Model file for the job. Use its own axes, mm. Face numbers are marked on the shaded views. A direction names the side the tool comes from. Give positions to 0.01 mm unless a question says otherwise; leave off trailing zeros. Order: outer loops, then holes, each group sorted by start corner. A loop starts at its lowest first (then second) coordinate and runs counter-clockwise, first axis right, second up. Notation, with made-up numbers: (44, 75) - (76, 75) arc R37 cw to (76, 111) - close; hole circle Ø5 at (65.5, 21.25). An arc over 180 degrees is marked (long way). Use CSV: the item, a comma, the result in double quotes. Start each with the question number.
(1) Drop flat-ended pins along their axis: pin 1 Ø2 at (y, z) = (35, 10.5) entering from -X; pin 2 Ø1.5 at (x, z) = (592, 18) entering from +Y; pin 3 Ø2 at (x, z) = (570, 10) entering from +Y. Give the stop position or say it passes through.
(2) Band-saw the part on C-C, the plane y = 49.5. Give the cut face in (x, z), then the cut area to 3 significant figures.
(3) Band-saw the part on D-D, the plane z = 10. Count the separate pieces of the cut face and the enclosed holes in it, then the cut area to 3 significant figures.
(4) Probe L1, parallel to Y at x = 582, z = 4.75; L2, parallel to Y at x = 574.5, z = 6.5; L3, parallel to Y at x = 594, z = 14. List the from-to ranges inside material, lowest first.
(5) Tool access for the marked faces 4, 5 and 6: list every direction of +Z, -Z, +X, -X, +Y, -Y with a clear straight run to the whole face (end or side of a thin tool).
(6) Band-saw the part on A-A, the plane x = 588. Give the cut face in (y, z), then the cut area to 3 significant figures.
(7) Pull direction Y, two halves, no side cores. Call the marked faces 1, 2 and 3: +Y half, -Y half, draft (parallel to the pull), parting line (faces both ways), or undercut.
(8) Band-saw the part on B-B, the plane y = 63. Give the cut face in (x, z), then the cut area to 3 significant figures.
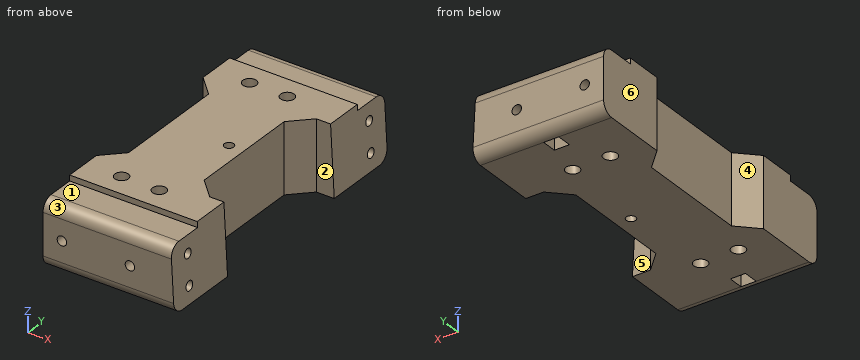
from build123d import *

# Parameters (mm, degrees)
CYLINDER445_R          = 1.25
CYLINDER445_DEPTH      = 20
BOX297_W               = 4
BOX297_H               = 4
BOX297_DEPTH           = 5
BOX298_W               = 4
BOX298_H               = 4
BOX298_DEPTH           = 5
CYLINDER444_R          = 1.25
CYLINDER444_DEPTH      = 15
CYLINDER443_R          = 1.25
CYLINDER443_DEPTH      = 15
CYLINDER442_R          = 1.25
CYLINDER442_DEPTH      = 15
CYLINDER441_R          = 1.25
CYLINDER441_DEPTH      = 15
CYLINDER450_R          = 1.8
CYLINDER450_DEPTH      = 18.5
CYLINDER451_R          = 1.8
CYLINDER451_DEPTH      = 18.5
CYLINDER446_R          = 1.8
CYLINDER446_DEPTH      = 18.5
CYLINDER447_R          = 1.8
CYLINDER447_DEPTH      = 18.5
CYLINDER449_R          = 1.25
CYLINDER449_DEPTH      = 15
CYLINDER448_R          = 1.25
CYLINDER448_DEPTH      = 15
CYLINDER440_R          = 1.25
CYLINDER440_DEPTH      = 15
CYLINDER439_R          = 1.25
CYLINDER439_DEPTH      = 15
BOX293_W               = 10
BOX293_H               = 82
BOX293_DEPTH           = 32
BOX293_PLACEMENT_ANGLE = 3
BOX300_W               = 35
BOX300_H               = 10
BOX300_DEPTH           = 1.5
BOX295_W               = 35
BOX295_H               = 20
BOX295_DEPTH           = 17
BOX292_W               = 35
BOX292_H               = 20
BOX292_DEPTH           = 17
BOX296_W               = 20
BOX296_H               = 40
BOX296_DEPTH           = 18.5
BOX299_W               = 35
BOX299_H               = 10
BOX299_DEPTH           = 1.5
FILLET107_R            = 3
CHAMFER030_SIZE        = 4.99


with BuildPart() as cylinder445:
    # Cylinder445 → Cylinder445 (new body)
    with BuildSketch(Plane(origin=(586, 31, 1.5), x_dir=(1, 0, 0), z_dir=(0, 0, 1))):
        Circle(CYLINDER445_R)
    extrude(amount=CYLINDER445_DEPTH)


with BuildPart() as box297:
    # Box297 → Box297 (new body)
    with BuildSketch(Plane(origin=(579, -6, 1.5), x_dir=(1, 0, 0), z_dir=(0, 0, 1))):
        with Locations((2, 2)):
            Rectangle(BOX297_W, BOX297_H)
    extrude(amount=BOX297_DEPTH)


with BuildPart() as fusion398:
    # Box298 → Box298 (new body)
    with BuildSketch(Plane(origin=(579, 64, 1.5), x_dir=(1, 0, 0), z_dir=(0, 0, 1))):
        with Locations((2, 2)):
            Rectangle(BOX298_W, BOX298_H)
    extrude(amount=BOX298_DEPTH)

    # Fusion398: union Box297
    add(box297.part)


with BuildPart() as cylinder444:
    # Cylinder444 → Cylinder444 (new body)
    with BuildSketch(Plane(origin=(585, 7, 6), x_dir=(0, 0, -1), z_dir=(1, 0, 0))):
        Circle(CYLINDER444_R)
    extrude(amount=CYLINDER444_DEPTH)


with BuildPart() as fusion396:
    # Cylinder443 → Cylinder443 (new body)
    with BuildSketch(Plane(origin=(585, 7, 14), x_dir=(0, 0, -1), z_dir=(1, 0, 0))):
        Circle(CYLINDER443_R)
    extrude(amount=CYLINDER443_DEPTH)

    # Fusion396: union Cylinder444
    add(cylinder444.part)


with BuildPart() as fusion396_1:
    # Fusion396 placement: moved
    add(fusion396.part.moved(Location((0, 58, 0))))


with BuildPart() as cylinder442:
    # Cylinder442 → Cylinder442 (new body)
    with BuildSketch(Plane(origin=(585, 7, 6), x_dir=(0, 0, -1), z_dir=(1, 0, 0))):
        Circle(CYLINDER442_R)
    extrude(amount=CYLINDER442_DEPTH)


with BuildPart() as fusion397:
    # Cylinder441 → Cylinder441 (new body)
    with BuildSketch(Plane(origin=(585, 7, 14), x_dir=(0, 0, -1), z_dir=(1, 0, 0))):
        Circle(CYLINDER441_R)
    extrude(amount=CYLINDER441_DEPTH)

    # Fusion395: union Cylinder442
    add(cylinder442.part)


with BuildPart() as fusion397_1:
    # Fusion395 placement: moved
    add(fusion397.part.moved(Location((0, -10, 0))))

    # Fusion397: union Fusion396
    add(fusion396_1.part)


with BuildPart() as cylinder450:
    # Cylinder450 → Cylinder450 (new body)
    with BuildSketch(Plane(origin=(584, 7, 10.5), x_dir=(1, 0, 0), z_dir=(0, 0, 1))):
        Circle(CYLINDER450_R)
    extrude(amount=CYLINDER450_DEPTH)


with BuildPart() as fusion403:
    # Cylinder451 → Cylinder451 (new body)
    with BuildSketch(Plane(origin=(584, 55, 10.5), x_dir=(1, 0, 0), z_dir=(0, 0, 1))):
        Circle(CYLINDER451_R)
    extrude(amount=CYLINDER451_DEPTH)

    # Fusion403: union Cylinder450
    add(cylinder450.part)


with BuildPart() as fusion403_1:
    # Fusion403 placement: moved
    add(fusion403.part.moved(Location((-9.5, 0, -9))))


with BuildPart() as cylinder446:
    # Cylinder446 → Cylinder446 (new body)
    with BuildSketch(Plane(origin=(584, 7, 10.5), x_dir=(1, 0, 0), z_dir=(0, 0, 1))):
        Circle(CYLINDER446_R)
    extrude(amount=CYLINDER446_DEPTH)


with BuildPart() as fusion405:
    # Cylinder447 → Cylinder447 (new body)
    with BuildSketch(Plane(origin=(584, 55, 10.5), x_dir=(1, 0, 0), z_dir=(0, 0, 1))):
        Circle(CYLINDER447_R)
    extrude(amount=CYLINDER447_DEPTH)

    # Fusion399: union Cylinder446
    add(cylinder446.part)


with BuildPart() as fusion405_1:
    # Fusion399 placement: moved
    add(fusion405.part.moved(Location((0.5, 0, -9))))

    # Fusion405: union Fusion403
    add(fusion403_1.part)


with BuildPart() as cylinder449:
    # Cylinder449 → Cylinder449 (new body)
    with BuildSketch(Plane(origin=(588, 71, 10), x_dir=(1, 0, 0), z_dir=(0, -1, 0))):
        Circle(CYLINDER449_R)
    extrude(amount=CYLINDER449_DEPTH)


with BuildPart() as fusion401:
    # Cylinder448 → Cylinder448 (new body)
    with BuildSketch(Plane(origin=(588, 6, 10), x_dir=(1, 0, 0), z_dir=(0, -1, 0))):
        Circle(CYLINDER448_R)
    extrude(amount=CYLINDER448_DEPTH)

    # Fusion401: union Cylinder449
    add(cylinder449.part)


with BuildPart() as fusion401_1:
    # Fusion401 placement: moved
    add(fusion401.part.moved(Location((-18, 0, 0))))


with BuildPart() as cylinder440:
    # Cylinder440 → Cylinder440 (new body)
    with BuildSketch(Plane(origin=(588, 71, 10), x_dir=(1, 0, 0), z_dir=(0, -1, 0))):
        Circle(CYLINDER440_R)
    extrude(amount=CYLINDER440_DEPTH)


with BuildPart() as fusion404:
    # Cylinder439 → Cylinder439 (new body)
    with BuildSketch(Plane(origin=(588, 6, 10), x_dir=(1, 0, 0), z_dir=(0, -1, 0))):
        Circle(CYLINDER439_R)
    extrude(amount=CYLINDER439_DEPTH)

    # Fusion394: union Cylinder440
    add(cylinder440.part)

    # Fusion404: union Fusion401
    add(fusion401_1.part)


with BuildPart() as box293:
    # Box293 → Box293 (new body)
    with BuildSketch(Plane.XY):
        with Locations((5, 41)):
            Rectangle(BOX293_W, BOX293_H)
    extrude(amount=BOX293_DEPTH)


with BuildPart() as box293_1:
    # Box293 placement: moved
    add(box293.part.moved(Location((600, -10, -3.6))).rotate(Axis((600, -10, -3.6), (0, -1, 0)), BOX293_PLACEMENT_ANGLE))


with BuildPart() as box300:
    # Box300 → Box300 (new body)
    with BuildSketch(Plane(origin=(565, 1, 18.5), x_dir=(1, 0, 0), z_dir=(0, 0, 1))):
        with Locations((17.5, 5)):
            Rectangle(BOX300_W, BOX300_H)
    extrude(amount=BOX300_DEPTH)


with BuildPart() as box295:
    # Box295 → Box295 (new body)
    with BuildSketch(Plane(origin=(565, 51, 1.5), x_dir=(1, 0, 0), z_dir=(0, 0, 1))):
        with Locations((17.5, 10)):
            Rectangle(BOX295_W, BOX295_H)
    extrude(amount=BOX295_DEPTH)


with BuildPart() as box292:
    # Box292 → Box292 (new body)
    with BuildSketch(Plane(origin=(565, -9, 1.5), x_dir=(1, 0, 0), z_dir=(0, 0, 1))):
        with Locations((17.5, 10)):
            Rectangle(BOX292_W, BOX292_H)
    extrude(amount=BOX292_DEPTH)


with BuildPart() as box296:
    # Box296 → Box296 (new body)
    with BuildSketch(Plane(origin=(570, 11, 1.5), x_dir=(1, 0, 0), z_dir=(0, 0, 1))):
        with Locations((10, 20)):
            Rectangle(BOX296_W, BOX296_H)
    extrude(amount=BOX296_DEPTH)


with BuildPart() as rear_cross_member_wide:
    # Box299 → Box299 (new body)
    with BuildSketch(Plane(origin=(565, 51, 18.5), x_dir=(1, 0, 0), z_dir=(0, 0, 1))):
        with Locations((17.5, 5)):
            Rectangle(BOX299_W, BOX299_H)
    extrude(amount=BOX299_DEPTH)

    # Fusion402: union Box300, Box295, Box292, Box296
    add(box300.part)
    add(box295.part)
    add(box292.part)
    add(box296.part)

    # Cut293: cut Box293
    add(box293_1.part, mode=Mode.SUBTRACT)

    # Cut294: cut Fusion404
    add(fusion404.part, mode=Mode.SUBTRACT)

    # Cut295: cut Fusion405
    add(fusion405_1.part, mode=Mode.SUBTRACT)

    # Fillet107
    fillet107_edges = [rear_cross_member_wide.edges().sort_by_distance(p)[0] for p in [
        (582.36636, 71, 1.5),
        (581.920894, 71, 18.5),
        (582.36636, -9, 1.5),
        (581.920894, -9, 18.5),
    ]]
    fillet(fillet107_edges, radius=FILLET107_R)

    # Chamfer030
    chamfer030_edges = [rear_cross_member_wide.edges().sort_by_distance(p)[0] for p in [
        (570, 51, 10.75),
        (590, 51, 10.75),
        (570, 11, 10.75),
        (590, 11, 10.75),
    ]]
    chamfer(chamfer030_edges, length=CHAMFER030_SIZE)

    # Cut296: cut Fusion397
    add(fusion397_1.part, mode=Mode.SUBTRACT)

    # Cut297: cut Fusion398
    add(fusion398.part, mode=Mode.SUBTRACT)

    # Cut298: cut Cylinder445
    add(cylinder445.part, mode=Mode.SUBTRACT)


solid = rear_cross_member_wide.part
Answer block:
1,pin 1,"stops at x = 570"
1,pin 2,"stops at y = 70.44"
1,pin 3,"stops at y = 56"
2,outline,"(566.51, 1.5) - (593.49, 1.5) - (593.49, 20) - (566.51, 20) - close"
2,area,"499 mm2"
3,separate pieces,"1"
3,enclosed holes,"5"
3,area,"2,030 mm2"
4,L1,"y = -9 to -6, -2 to 64, 68 to 71"
4,L2,"y = -9 to 5.2, 8.8 to 53.2, 56.8 to 71"
4,L3,"y = -9 to -4.25, -1.75 to 11.99, 50.01 to 63.75, 66.25 to 71"
5,face 4,"+Z, -Z, -X"
5,face 5,"+Z, -Z, +X"
5,face 6,"+Z, -Z, -X, +Y, -Y"
6,outline,"(-9, 4.5) arc R3 ccw to (-6, 1.5) - (68, 1.5) arc R3 ccw to (71, 4.5) - (71, 8.75) - (56, 8.75) - (56, 11.25) - (71, 11.25) - (71, 15.5) arc R3 ccw to (68, 18.5) - (61, 18.5) - (61, 20) - (1, 20) - (1, 18.5) - (-6, 18.5) arc R3 ccw to (-9, 15.5) - (-9, 11.25) - (6, 11.25) - (6, 8.75) - (-9, 8.75) - close; hole circle Ø2.5 at (-3, 6); hole circle Ø2.5 at (-3, 14); hole circle Ø2.5 at (65, 6); hole circle Ø2.5 at (65, 14)"
6,area,"1,350 mm2"
7,face 1,"draft"
7,face 2,"undercut"
7,face 3,"-Y half"
8,outline,"(565, 1.5) - (599.73, 1.5) - (598.84, 18.5) - (565, 18.5) - close; hole circle Ø2.5 at (570, 10); hole circle Ø2.5 at (588, 10)"
8,area,"573 mm2"
